```python
from build123d import *

# Parameters (mm, degrees)
BOSS_EXTRUDE1_DEPTH = 10.16
CUT_EXTRUDE1_REACH  = 48.698
SKETCH3_W           = 50.546
SKETCH3_H           = 20.972046169
BOSS_EXTRUDE2_DEPTH = 5.08
CUT_EXTRUDE2_REACH  = 65.84
FILLET1_R           = 5.08
FILLET2_R           = 3.81
FILLET3_R           = 1.27
SKETCH5_R           = 1.5999968
CUT_EXTRUDE3_DEPTH  = 44.788596105


with BuildPart() as part:
    # Sketch1 → Boss-Extrude1 (new body)
    with BuildSketch(Plane(origin=(0, 0, 0), x_dir=(1, 0, 0), z_dir=(0, 1, 0))):
        with BuildLine():
            Line((-15.113, 0), (-15.113, -25.4))
            Line((-15.113, -25.4), (15.113, -25.4))
            Line((15.113, -25.4), (15.113, -3.81))
            Line((15.113, -3.81), (22.733, -3.81))
            Line((22.733, -3.81), (22.733, 0))
            Line((22.733, 0), (15.113, 0))
            Line((15.113, 0), (11.303, 0))
            ThreePointArc((11.303, 0), (-11.136399388, -1.933498813), (10.641508775, 3.81))
            Line((10.641508775, 3.81), (22.733, 3.81))
            Line((22.733, 3.81), (22.733, 7.62))
            Line((22.733, 7.62), (13.051374219, 7.62))
            ThreePointArc((13.051374219, 7.62), (-3.946983052, 14.588491827), (-15.113, 0))
        make_face()
    extrude(amount=BOSS_EXTRUDE1_DEPTH)

    # Sketch2 → Cut-Extrude1 (cut, up to next)
    with BuildSketch(Plane.ZY.offset(15.113), mode=Mode.PRIVATE) as cut_extrude1_sk1:
        Polygon((25.4, 10.16), (21.70206242, 0), (25.4, 0), align=None)
    cut_extrude1_tool1 = extrude(cut_extrude1_sk1.sketch, amount=-CUT_EXTRUDE1_REACH, mode=Mode.PRIVATE) & part.part
    add(cut_extrude1_tool1.solids().sort_by_distance((-15.113, 3.386667, 24.167354))[0], mode=Mode.SUBTRACT)

    # Sketch3 → Boss-Extrude2 (add)
    with BuildSketch(Plane(origin=(0, -6.974908414, 19.16340337), x_dir=(1, 0, 0), z_dir=(0, -0.34202014332566916, 0.9396926207859082))):
        with Locations((0, 17.908565583)):
            Rectangle(SKETCH3_W, SKETCH3_H)
    extrude(amount=BOSS_EXTRUDE2_DEPTH)

    # Sketch4 → Cut-Extrude2 (cut, up to next)
    with BuildSketch(Plane.ZY.offset(25.273), mode=Mode.PRIVATE) as cut_extrude2_sk1:
        Polygon((27.108085504, 0), (26.475700933, -1.737462328), (21.70206242, 0), align=None)
    cut_extrude2_tool1 = extrude(cut_extrude2_sk1.sketch, amount=-CUT_EXTRUDE2_REACH, mode=Mode.PRIVATE) & part.part
    add(cut_extrude2_tool1.solids().sort_by_distance((-25.273, -0.579154, 25.095283))[0], mode=Mode.SUBTRACT)

    # Fillet1
    fillet1_edges = [part.edges().sort_by_distance(p)[0] for p in [
        (-15.113, 5.08, 23.55103121),
        (15.113, 5.08, 23.55103121),
        (0, 10.16, 25.4),
    ]]
    fillet(fillet1_edges, radius=FILLET1_R)

    # Fillet2
    fillet2_edges = [part.edges().sort_by_distance(p)[0] for p in [
        (13.051374219, 5.08, -7.62),
    ]]
    fillet(fillet2_edges, radius=FILLET2_R)

    # Fillet3
    fillet3_edges = [part.edges().sort_by_distance(p)[0] for p in [
        (15.113, 5.08, 3.81),
    ]]
    fillet(fillet3_edges, radius=FILLET3_R)

    # Sketch5 → Cut-Extrude3 (cut, through all)
    with BuildSketch(Plane.XY.offset(3.81)):
        with Locations((19.558, 5.08)):
            Circle(SKETCH5_R)
    extrude(amount=-CUT_EXTRUDE3_DEPTH, mode=Mode.SUBTRACT)


solid = part.part
```
Source: CAD feature listing. Evaluate the final solid. Frame: model axes, mm. A direction names the side the tool comes from. Round coordinates to 2 decimals unless told otherwise and drop trailing zeros. Loops run counter-clockwise (first coordinate to the right, second up) from the corner with the lowest first, then second, coordinate; pieces in that order, holes last.
1. Mould query, pull axis Z, two halves, no side actions, for faces 5 (the flat face through (3.4, 10.16, 11.3)), 6 (the cylindrical face through (-16.64, 6.27, 22.44)), 7 (the flat face through (21, 4, 3.81)). Classes: released by +Z, released by -Z, zero draft, split by the parting line, or undercut.
2. Section query B-B on z = 1. Output: boundary loops of the cut face in (x, y), and give its area (3 significant figures).
3. Contact query for flat-ended pins moving along their axis: pin 1 (1.5 mm diameter, centred on x = -20, y = 10.5, fed in from -Z); pin 2 (1.1 mm diameter, centred on y = 5.5, z = 2, fed in from +X); pin 3 (5 mm diameter, centred on x = -12, z = 12, fed in from +Y); pin 4 (5 mm diameter, centred on y = 13.5, z = 6, fed in from -X). Output: stop coordinate, or through.
4. Access query for faces 1 (the flat face through (17, 5, 0)), 2 (the cylindrical face through (21.036, 4.467, -5.688)), 3 (the flat face through (22.733, 5, -6)), 4 (the flat face through (-0.354, 14.371, 26.933)). Directions: +Z, -Z, +X, -X, +Y, -Y. A direction counts if a zero-diameter tool reaches every point of the face in a straight line with its end or side. Return the directions, or none.
5. Section query D-D on x = -10.5. Output: boundary loops of the cut face in (y, z), and give its area (3 significant figures).
6. Section query A-A on x = 0. Output: boundary loops of the cut face in (y, z).
7. Ray query, L1, parallel to Z at x = 18, y = 7.75; L2, parallel to Y at x = 0, z = -12.5; L3, parallel to Z at x = 0, y = 6.5. Return the intervals inside material, ascending.
8. Section query C-C on y = 5.08. Give the number of separate pieces and of enclosed holes in the cut face, and give its area (3 significant figures).
Answers below:
1. face 5: zero draft
1. face 6: released by -Z
1. face 7: undercut
2. outline: (-15.11, 0) - (-11.26, 0) - (-11.26, 10.16) - (-15.11, 10.16) - close; (11.26, 0) - (22.73, 0) - (22.73, 10.16) - (11.26, 10.16) - close; hole circle Ø3.2 at (19.56, 5.08)
2. area: 148 mm2
3. pin 1: stops at z = 25.24
3. pin 2: stops at x = 22.73
3. pin 3: stops at y = 10.16
3. pin 4: passes through
4. face 1: +X, +Y, -Y
4. face 2: -Z
4. face 3: -Z, +X, +Y, -Y
4. face 4: +Y
5. outline: (0, -10.87) - (10.16, -10.87) - (10.16, -4.18) - (0, -4.18) - close; (0, 4.18) - (10.16, 4.18) - (10.16, 21.84) arc R5.08 cw to (13.5, 26.62) - (19.71, 28.87) - (17.97, 33.65) - (0, 27.11) - close
5. area: 369 mm2
6. outline: (0, -15.11) - (10.16, -15.11) - (10.16, -11.3) - (0, -11.3) - close; (0, 11.3) - (10.16, 11.3) - (10.16, 21.84) arc R5.08 cw to (13.5, 26.62) - (19.71, 28.87) - (17.97, 33.65) - (0, 27.11) - close
7. L1: z = -7.62 to -3.81, 0 to 3.81, 23.99 to 29.93
7. L2: y = 0 to 10.16
7. L3: z = -15.11 to -11.3, 11.3 to 29.47
8. separate pieces: 3
8. enclosed holes: 0
8. area: 979 mm2
